Autodesk Inventor part; units mm, degrees
ref_plane "YZ Plane" through (0, 0, 0) normal (1, 0, 0) x (0, 1, 0)
ref_plane "XZ Plane" through (0, 0, 0) normal (0, 1, 0) x (-1, 0, 0)
ref_plane "XY Plane" through (0, 0, 0) normal (0, 0, 1) x (1, 0, 0)
sketch "Sketch2" plane through (0, 0, 0) normal (0, 1, 0) x (-1, 0, 0)
  line L0 (6.5, 0) -> (6.5, 5)
  line L1 (6.5, 5) -> (5, 5)
  line L2 (6.5, 5) -> (6.5, 0)
  line L3 (0, -1) -> (0, 6)
  line L4 (6.5, 0) -> (2, 0)
  line L5 (2, 0) -> (1, 1)
  line L6 (1, 1) -> (1, 1.5)
  line L7 (5, 5) -> (1, 1.5)
  point P0 (0, 0)
  dimension "d4" = 5
  dimension "d5" = 1.5
  dimension "d11" = 6.5
  dimension "d26" = 4.5
  dimension "d27" = 0.5
  dimension "d28" = 1
  dimension "d29" = 2
  dimension "d31" = 1
revolve "Revolution2" add sketch "Sketch2" angle 360 about axis through (0, 0, -10) along (0, 0, 1)
fillet "Fillet4" radius 0.2 2 edges at (1, 0, 1) (1, 0, 1.5)
properties part number "nozzle_big" material "Glass"
Verification items for the finished model (mm, model axes). Round coordinates to 2 decimals unless told otherwise and drop trailing zeros. Order: outer loops, then holes, each group sorted by start corner. A loop starts at its lowest first (then second) coordinate and runs counter-clockwise, first axis right, second up. Notation, with made-up numbers: (30, 85) - (85, 85) arc R19 cw to (85, 118) - close; hole circle Ø9 at (44, -14.75). An arc over 180 degrees is marked (long way). Use CSV: the item, a comma, the result in double quotes. Start each with the question number.
1) Thickness scan on L1, parallel to X at y = 0, z = 1.25; L2, parallel to X at y = -1, z = 3.85. Record the ranges inside material, lowest first.
2) Section check B-B, the plane y = 5.5. Record the cut outline in (x, z), plus the area to 3 significant figures.
3) Section check C-C, the plane z = 4.4. Record the cut outline in (x, y).
4) Section check A-A, the plane z = 1.25. Record the cut outline in (x, y), plus the area to 3 significant figures.
5) Mould release check, pull along Y, two halves, no side actions. Record for faces 1 (the conical face through (-1.25, -0.39, 1.77)), 2 (the cylindrical face through (5.158, 3.955, 2.535)), 3 (the flat face through (-2, 5, 5)): +Y half, -Y half, draft (parallel to the pull), parting line (faces both ways), or undercut.
6) Go/stop test with flat-tipped pins: P1, Ø2, axis at y = -4.5, z = 2, coming from the +X side; P2, Ø3, axis at x = 0, y = 0, coming from the +Z side. Record where each tip stops, or that it passes through.
Answers:
1,L1,"x = -6.5 to -1, 1 to 6.5"
1,L2,"x = -6.42 to -3.55, 3.55 to 6.42"
2,outline,"(-3.46, 0) - (3.46, 0) - (3.46, 5) - (-3.46, 5) - close"
2,area,"34.6 mm²"
3,outline,"circle Ø13 at (0, 0); hole circle Ø8.63 at (0, 0)"
4,outline,"circle Ø13 at (0, 0); hole circle Ø2 at (0, 0)"
4,area,"130 mm²"
5,face 1,"undercut"
5,face 2,"parting line"
5,face 3,"draft"
6,P1,"stops at x = 5.48"
6,P2,"stops at z = 1.94"
